Here's how the part is built. I have some questions about the finished solid (model axes, mm). Face numbers are marked on the shaded views. A direction names the side the tool comes from. Coordinates: 2 decimals unless noted, no trailing zeros. Write each loop counter-clockwise with the first axis right and the second up, starting at its lowest first coordinate (ties: lowest second). Pieces come first, ordered by that corner, then holes. Notation, with made-up numbers: (52, 22.5) -> (87, 22.5) arc R28 cw to (87, 60.5) -> close; hole circle Ø11 at (83, 84). An arc over 180 degrees is marked (long way). Use a Markdown table: item, result. Add a question column.
```python
from build123d import *

# Parameters (mm, degrees)
BOSS_EXTRU_1_DEPTH                = 23
DIAM_TRE_DU_PER_AGE_2_0_2_1_D     = 2
DIAM_TRE_DU_PER_AGE_2_0_2_1_DEPTH = 3
ESQUISSE4_W                       = 15
ESQUISSE4_H                       = 15
BOSS_EXTRU_3_DEPTH                = 2
ESQUISSE6_W                       = 15
ESQUISSE6_H                       = 15
ESQUISSE6_W_2                     = 4
ESQUISSE6_H_2                     = 12
BOSS_EXTRU_4_DEPTH                = 3


with BuildPart() as part:
    # Esquisse1 → Boss.-Extru.1 (new body)
    with BuildSketch(Plane.XY):
        with BuildLine():
            Line((-5, 2.291287847), (-5, -2.291287847))
            ThreePointArc((-5, -2.291287847), (5.5, 0), (-5, 2.291287847))
        make_face()
        with BuildLine():
            Line((-2, 1.5), (-2, -1.5))
            ThreePointArc((-2, -1.5), (2.5, 0), (-2, 1.5))
        make_face(mode=Mode.SUBTRACT)
    extrude(amount=BOSS_EXTRU_1_DEPTH)

    # Diamètre du perçage Ø2.0 (2)1
    with Locations(Plane(origin=(-5, -0.001287847, 3.5), x_dir=(0, 0, -1), z_dir=(-1, 0, 0))):
        with Locations((0, 0), (-8, 0)):
            Hole(DIAM_TRE_DU_PER_AGE_2_0_2_1_D / 2, depth=DIAM_TRE_DU_PER_AGE_2_0_2_1_DEPTH)

    # Esquisse4 → Boss.-Extru.3 (add)
    with BuildSketch(Plane.XY.offset(23)):
        Rectangle(ESQUISSE4_W, ESQUISSE4_H)
    extrude(amount=BOSS_EXTRU_3_DEPTH)

    # Esquisse6 → Boss.-Extru.4 (add)
    with BuildSketch(Plane.XY.offset(25)):
        Rectangle(ESQUISSE6_W, ESQUISSE6_H)
        Rectangle(ESQUISSE6_W_2, ESQUISSE6_H_2, mode=Mode.SUBTRACT)
    extrude(amount=BOSS_EXTRU_4_DEPTH)


solid = part.part
```
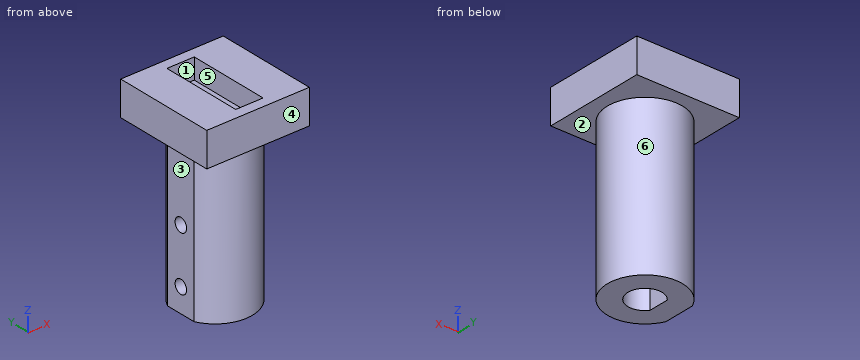
Q1. Which directions (+Z, -Z, +X, -X, +Y, -Y) give clear straight access to the entire face, cutting with the end or side of a thin tool? Please do the marked faces 4, 5 and 6.
Q2. Suppose I cut it at C-C, the plane z = 3.5. Write out the boundary of the cut face in (x, y).
Q3. Suppose I cut it at B-B, the plane y = 5. Write out the boundary of the cut face in (x, z).
Q4. Suppose I cut it at D-D, the plane x = 0. Write out the boundary of the cut face in (y, z), and give its area (3 significant figures).
Q5. Will these pins go through, and if not, where does the flat tip stop? pin 1 (3 mm diameter, centred on y = 0, z = 3.5, fed in from +X); pin 2 (8 mm diameter, centred on x = -1.5, z = 13, fed in from -Y); pin 3 (5 mm diameter, centred on y = 0, z = 13.5, fed in from -X).
Q6. Thinking about a two-plate mould opening in X: for the marked faces 1, 2 and 3, which applies, released by +X, released by -X, zero draft, split by the parting line, or undercut?
Q7. Suppose I cut it at A-A, the plane x = 5. Write out the boundary of the cut face in (y, z).
Q8. Please list where these lines run through material, in increasing order: line 1 (Z direction, x = -4, y = 0); line 2 (X direction, y = 0, z = 10.75); line 3 (Z direction, x = 6.25, y = -3.75).
Answer key:
| question | item | result |
|---|---|---|
| 1 | face 4 | +Z, -Z, +X, -X, -Y |
| 1 | face 5 | +Z |
| 1 | face 6 | -Z |
| 2 | outline | (-5, -2.29) arc R5.5 ccw (long way) to (-5, 2.29) -> (-5, 1) -> (-2, 1) -> (-2, 1.5) arc R2.5 cw (long way) to (-2, -1.5) -> (-2, -1) -> (-5, -1) -> close |
| 3 | outline | (-7.5, 23) -> (-2.29, 23) -> (-2.29, 0) -> (2.29, 0) -> (2.29, 23) -> (7.5, 23) -> (7.5, 28) -> (2, 28) -> (2, 25) -> (-2, 25) -> (-2, 28) -> (-7.5, 28) -> close |
| 4 | outline | (-7.5, 23) -> (-5.5, 23) -> (-5.5, 0) -> (-2.5, 0) -> (-2.5, 23) -> (2.5, 23) -> (2.5, 0) -> (5.5, 0) -> (5.5, 23) -> (7.5, 23) -> (7.5, 28) -> (6, 28) -> (6, 25) -> (-6, 25) -> (-6, 28) -> (-7.5, 28) -> close |
| 4 | area | 177 mm^2 |
| 5 | pin 1 | stops at x = 5.5 |
| 5 | pin 2 | stops at y = -5.5 |
| 5 | pin 3 | stops at x = -5 |
| 6 | face 1 | undercut |
| 6 | face 2 | zero draft |
| 6 | face 3 | released by -X |
| 7 | outline | (-7.5, 23) -> (-2.29, 23) -> (-2.29, 0) -> (2.29, 0) -> (2.29, 23) -> (7.5, 23) -> (7.5, 28) -> (-7.5, 28) -> close |
| 8 | line 1 | z = 0 to 2.5, 4.5 to 10.5, 12.5 to 28 |
| 8 | line 2 | x = 2.5 to 5.5 |
| 8 | line 3 | z = 23 to 28 |
